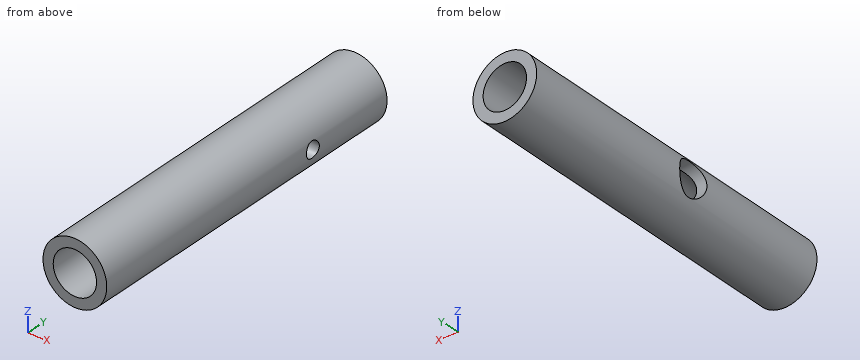
Autodesk Inventor part; units mm, degrees
ref_plane "YZ Plane" through (0, 0, 0) normal (1, 0, 0) x (0, 1, 0)
ref_plane "XZ Plane" through (0, 0, 0) normal (0, 1, 0) x (-1, 0, 0)
ref_plane "XY Plane" through (0, 0, 0) normal (0, 0, 1) x (1, 0, 0)
sketch "Sketch1" plane through (0, 0, 0) normal (0, 1, 0) x (-1, 0, 0)
  circle A0 centre (0, 0) radius 1.0795
  circle A1 centre (0, 0) radius 1.5875
  dimension "d0" = 2.159
  dimension "d1" = 3.175
extrude "Extrusion1" add sketch "Sketch1" along normal blind 17.272
sketch "Sketch2" plane through (0, 0, 0) normal (1, 0, 0) x (0, 1, 0)
  circle A0 centre (7.62, 0) radius 0.8382
  line L0 (17.272, -1.5875) -> (17.272, 1.5875)
  circle A1 centre (12.7, 0) radius 0.3969
  line L1 (17.272, 1.0795) -> (17.272, -1.0795)
  point P0 (0, 0)
  dimension "d4" = 1.6764
  dimension "d5" = 9.652
  dimension "d8" = 0.7937
  dimension "d9" = 4.572
extrude "Extrusion2" cut sketch "Sketch2" against normal blind 17.272 contours A0
extrude "Extrusion3" cut sketch "Sketch2" along normal blind 25.4 contours A1
properties part number "Valve Tube"
For this review, take the finished solid that the model builds, in its own axes (mm). Give positions to 0.01 mm unless a question says otherwise; leave off trailing zeros. Loops run counter-clockwise (first coordinate to the right, second up) from the corner with the lowest first, then second, coordinate; pieces in that order, holes last. Notation, with made-up numbers: M 41,14 L 49,14 A14 ccw 49,18 Z; hole C 16,-36 d2. An arc over 180 degrees is marked long. Put each result on its own line as item: value. Start each with the question number.
(1) Add section D-D, the plane x = 1.3. Write out the cut boundary in (y, z), then the cut area to 3 significant figures.
(2) Add section A-A, the plane x = 0. Write out the cut boundary in (y, z), then the cut area to 3 significant figures.
(3) For pin 1 (1.5 mm diameter, centred on x = -1, y = 9.5, fed in from +Z), flat-tipped, find the tip position at first contact; note if it passes through.
(4) Wall thickness on L1, parallel to X at y = 11.75, z = -0.05; L2, parallel to Y at x = -1.35, z = -0.05; L3, parallel to Z at x = 0.6, y = 3: over which ranges is each line inside the solid? List them lowest first.
(5) Add section B-B, the plane z = 0. Write out the cut boundary in (x, y).
(6) Add section C-C, the plane y = 15.5. Write out the cut boundary in (x, z) (1 decimal).
Result:
1. outline: M 0,-0.91 L 17.27,-0.91 L 17.27,0.91 L 0,0.91 Z; hole C 12.7,0 d0.79
1. area: 31.0 mm^2
2. outline: M 0,-1.59 L 17.27,-1.59 L 17.27,-1.08 L 0,-1.08 Z; M 0,1.08 L 17.27,1.08 L 17.27,1.59 L 0,1.59 Z
2. area: 17.5 mm^2
3. pin 1: stops at z = 1.57
4. L1: x = -1.59 to -1.08, 1.08 to 1.59
4. L2: y = 0 to 6.78, 8.46 to 17.27
4. L3: z = -1.47 to -0.9, 0.9 to 1.47
5. outline: M -1.59,0 L -1.08,0 L -1.08,6.78 L -1.59,6.78 Z; M -1.59,8.46 L -1.08,8.46 L -1.08,17.27 L -1.59,17.27 Z; M 1.08,0 L 1.59,0 L 1.59,12.3 L 1.08,12.3 Z; M 1.08,13.1 L 1.59,13.1 L 1.59,17.27 L 1.08,17.27 Z
6. outline: C 0,0 d3.2; hole C 0,0 d2.2
